Check sheet for the drawn part. Datum: minimum x, y, z corner. Units: mm. A direction names the side the tool comes from. Coordinates: 2 decimals unless noted, no trailing zeros. Write each loop counter-clockwise with the first axis right and the second up, starting at its lowest first coordinate (ties: lowest second). Pieces come first, ordered by that corner, then holes. Notation, with made-up numbers: (47, -19.75) - (56, -19.75) arc R20 cw to (56, 17.25) - close; hole circle Ø11 at (63.25, 22.25). An arc over 180 degrees is marked (long way). Use one line per item in the form item = value. Start each with the question number.
1. Go/stop test with flat-tipped pins: pin 1 Ø2.5 at (x, y) = (1, 32.5) entering from -Z; pin 2 Ø2.5 at (x, z) = (1, 3.5) entering from +Y; pin 3 Ø2 at (x, y) = (8, 10.5) entering from -Z. Record where each tip stops, or that it passes through.
2. Cross-section at C-C on y = 30.5. Record the boundary of the cut face in (x, z).
3. Cross-section at A-A on y = 24. Record the boundary of the cut face in (x, z).
4. Scan lines: line 1 along X through (y, z) = (10.5, 21.5); line 2 along X through (y, z) = (3.5, 18.5); line 3 along Z through (x, y) = (14.25, 10). Record each from-to range of solid material in increasing order.
5. Cross-section at B-B on z = 5.5. Record the boundary of the cut face in (x, y).
6. Draft check along Y on the marked faces 1, 2 and 3. Enter one of: +Y half, -Y half, draft (parallel to the pull), parting line (faces both ways), or undercut.
7. Tool access check on the marked faces 4, 5 and 6. Record the directions out of +Z, -Z, +X, -X, +Y, -Y that give a thin tool (end or side, any length) a straight path to the whole face; none if there is none.
8. Cross-section at D-D on x = 25.25. Record the boundary of the cut face in (y, z), then the cut area to 3 significant figures.
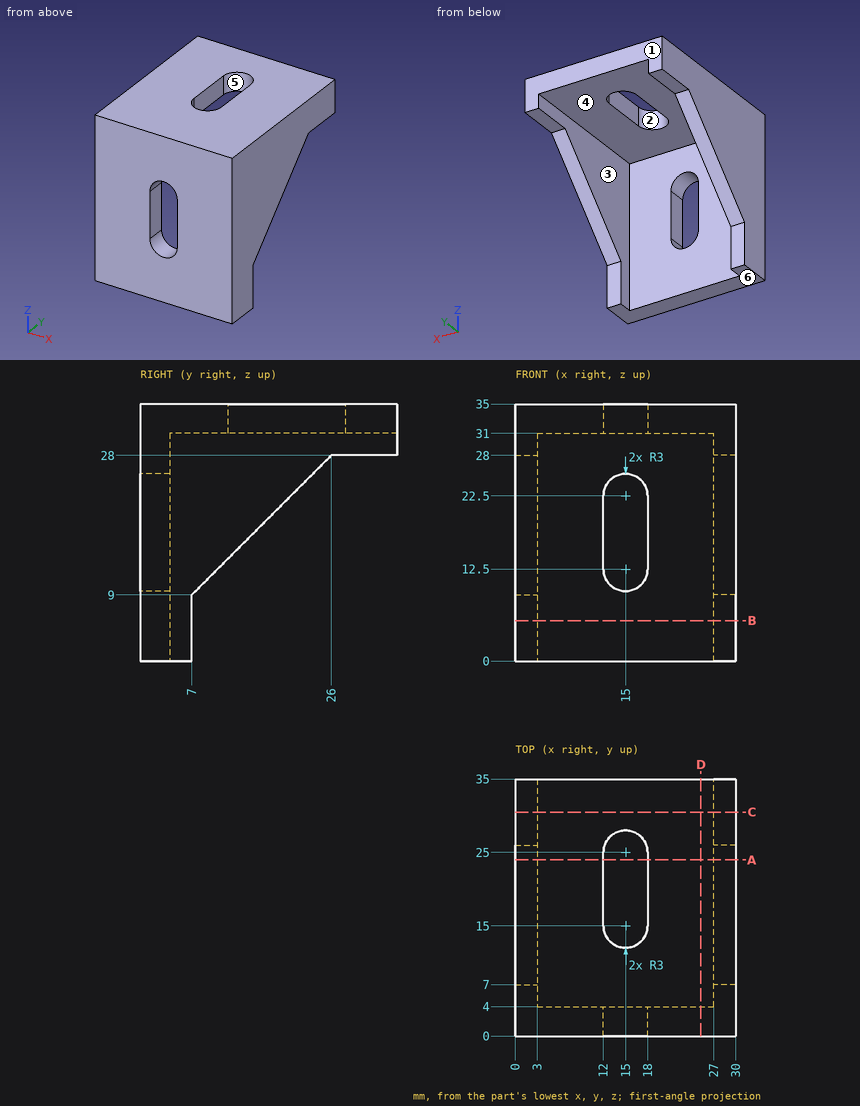
Final values:
q1.pin_1 = 28
q1.pin_2 = 7
q1.pin_3 = 31
q2.outline = (0, 28) - (3, 28) - (3, 31) - (27, 31) - (27, 28) - (30, 28) - (30, 35) - (0, 35) - close
q3.outline = (0, 26) - (3, 26) - (3, 31) - (12, 31) - (12, 35) - (0, 35) - close; (18, 31) - (27, 31) - (27, 26) - (30, 26) - (30, 35) - (18, 35) - close
q4.line_1 = 0 to 3, 27 to 30
q4.line_2 = 0 to 12, 18 to 30
q4.line_3 = 31 to 35
q5.outline = (0, 0) - (30, 0) - (30, 7) - (27, 7) - (27, 4) - (3, 4) - (3, 7) - (0, 7) - close
q6.face_1 = +Y half
q6.face_2 = undercut
q6.face_3 = draft
q7.face_4 = -Z, +Y
q7.face_5 = +Z, -Z
q7.face_6 = -Z, +X, -X, +Y, -Y
q8.outline = (0, 0) - (4, 0) - (4, 31) - (35, 31) - (35, 35) - (0, 35) - close
q8.area = 264 mm²
